from build123d import *

# Parameters (mm, degrees)
SKETCH_1_W               = 64
SKETCH_1_H               = 34
SKETCH_1_W_2             = 60
SKETCH_1_H_2             = 30
EXTRUDE_1_DEPTH          = 28
SKETCH_1_2_W             = 60
SKETCH_1_2_H             = 30
EXTRUDE_1_2_DEPTH        = 2
FILLET_3_R               = 2.5
CUT_EXTRUDE_6_DEPTH      = 55.442630355
CUT_EXTRUDE_6_DEPTH_BACK = 55.442630355
FILLET_4_R               = 10
SKETCH_8_W               = 30
SKETCH_8_H               = 4.631369762
CUT_EXTRUDE_7_DEPTH      = 71.121323433
CUT_EXTRUDE_9_DEPTH      = 45.598206242
CUT_EXTRUDE_9_DEPTH_BACK = 45.598206242
SKETCH_9_R               = 2


with BuildPart() as part:
    # Эскиз1 → Extrude 1 (new body)
    with BuildSketch(Plane(origin=(0, 0, 0), x_dir=(1, 0, 0), z_dir=(0, 1, 0))):
        Rectangle(SKETCH_1_W, SKETCH_1_H)
        Rectangle(SKETCH_1_W_2, SKETCH_1_H_2, mode=Mode.SUBTRACT)
    extrude(amount=EXTRUDE_1_DEPTH)

    # Эскиз1<2> → Extrude 1 2 (add)
    with BuildSketch(Plane(origin=(0, 0, 0), x_dir=(1, 0, 0), z_dir=(0, 1, 0))):
        Rectangle(SKETCH_1_2_W, SKETCH_1_2_H)
    extrude(amount=EXTRUDE_1_2_DEPTH)

    # Скругление3
    fillet_3_edges = [part.edges().sort_by_distance(p)[0] for p in [
        (-30, 15, -15),
        (-30, 15, 15),
        (-32, 14, -17),
        (-32, 14, 17),
    ]]
    fillet(fillet_3_edges, radius=FILLET_3_R)

    # Эскиз3 → Вырез-Вытянуть6 (cut, two sides: drawn at the far end of the back side and taken through both)
    with BuildSketch(Plane.XY.offset(17).offset(-CUT_EXTRUDE_6_DEPTH_BACK)):
        Polygon((-13, 28), (32, 7), (32, 28), align=None)
    extrude(amount=CUT_EXTRUDE_6_DEPTH + CUT_EXTRUDE_6_DEPTH_BACK, mode=Mode.SUBTRACT)

    # Скругление4
    # the kernel refuses this fillet: 10 mm, written as the material it takes off along each edge
    with BuildSketch(Plane(origin=(32, 7, -32.921575595), x_dir=(0, -1, 0), z_dir=(0, 0, 1))) as fillet_4_piece_1:
        with BuildLine():
            CenterArc((FILLET_4_R * 0.636863023816, -FILLET_4_R), FILLET_4_R, 90, 64.983106522)
            Line((-FILLET_4_R * 0.269320116179, -FILLET_4_R * 0.577114534669), (0, 0))
            Line((0, 0), (FILLET_4_R * 0.636863023816, 0))
        make_face()
    extrude(amount=65.843151191, mode=Mode.SUBTRACT)
    with BuildSketch(Plane(origin=(-13, 28, 22.546233419), x_dir=(0.9061831399952657, -0.4228854653311234, 0), z_dir=(0, 0, -1)), Plane(origin=(-13, 28, -9.453766581), x_dir=(0.9061831399952657, -0.4228854653311234, 0), z_dir=(0, 0, -1))) as fillet_4_piece_2:
        with BuildLine():
            CenterArc((FILLET_4_R * 0.22184933675, FILLET_4_R), FILLET_4_R, 244.983106522, 25.016893478)
            Line((-FILLET_4_R * 0.201036128582, FILLET_4_R * 0.0938168600047), (0, 0))
            Line((0, 0), (FILLET_4_R * 0.22184933675, 0))
        make_face()
    extrude(amount=13.092466837, mode=Mode.SUBTRACT)

    # Эскиз8 → Вырез-Вытянуть7 (cut, through all)
    with BuildSketch(Plane.ZY.offset(-30)):
        with Locations((0, 4.315684881)):
            Rectangle(SKETCH_8_W, SKETCH_8_H)
    extrude(amount=-CUT_EXTRUDE_7_DEPTH, mode=Mode.SUBTRACT)

    # Эскиз9 → Вырез-Вытянуть9 (cut, two sides: drawn at the far end of the back side and taken through both)
    with BuildSketch(Plane(origin=(0, 2, 0), x_dir=(1, 0, 0), z_dir=(0, 1, 0)).offset(-CUT_EXTRUDE_9_DEPTH_BACK)):
        with Locations(Location((-22.5, -10, 0), (0, 0, 270))):
            Circle(SKETCH_9_R)
        with Locations(Location((-22.5, 10, 0), (0, 0, 270))):
            Circle(SKETCH_9_R)
        with Locations(Location((22.5, 10, 0), (0, 0, 270))):
            Circle(SKETCH_9_R)
        with Locations(Location((22.5, -10, 0), (0, 0, 270))):
            Circle(SKETCH_9_R)
    extrude(amount=CUT_EXTRUDE_9_DEPTH + CUT_EXTRUDE_9_DEPTH_BACK, mode=Mode.SUBTRACT)


solid = part.part
Part model, mm, in its own coordinate system. A direction names the side the tool comes from. Round coordinates to 2 decimals unless told otherwise and drop trailing zeros. Write each loop counter-clockwise with the first axis right and the second up, starting at its lowest first coordinate (ties: lowest second). Pieces come first, ordered by that corner, then holes. Notation, with made-up numbers: M 41,61.5 L 96,61.5 A15 cw 96,70.5 Z; hole C 40,66 d10. An arc over 180 degrees is marked long. Return JSON: item names as keys, results as strings. Group by question number.
(1) Saw through at B-B on x = -22.5. Write the cut outline in (y, z), then the cut area to 3 significant figures.
(2) Saw through at D-D on y = 15.75. Write the cut outline in (x, z).
(3) Pin check, flat tip, straight feed: pin 1 Ø15 at (x, z) = (2.5, -4) entering from +Y. Stop position of the tip, or through.
(4) Saw through at C-C on z = -5.5. Write the cut outline in (x, y), then the cut area to 3 significant figures.
(5) Which spindle directions (+Z, -Z, +X, -X, +Y, -Y) get a long thin tool onto all of the face, cutting with end or side? Do faces 1 (the face through (-30.5, 28, -0.1)), 2 (the face through (-29.248, 15.182, -14.287)). Say none if no direction does.
(6) Drill centre lines: probe 1 along X at (y, z) = (0.4, 10); probe 2 along Z at (x, y) = (-22.5, 1.05); probe 3 along Z at (x, y) = (3, 19.5). Where is each one in solid material? Low to high.
(7) Saw through at A-A on z = -10. Write the cut outline in (x, y), then the cut area to 3 significant figures.
(8) Two-plate mould, pull along Z, no slides. Class faces 3 (the face through (-13.08, 27.77, -15.99)), 4 (the face through (-31.287, 14.196, 16.248)), 5 (the face through (-20.517, 0.986, 9.74)): +Z half, -Z half, draft (parallel to the pull), parting line (faces both ways), or undercut.
Returned:
{
 "1": {"outline": "M 0,-17 L 28,-17 L 28,-15 L 2,-15 L 2,-12 L 0,-12 Z; M 0,-8 L 2,-8 L 2,8 L 0,8 Z; M 0,12 L 2,12 L 2,15 L 28,15 L 28,17 L 0,17 Z", "area": "156 mm²"},
 "2": {"outline": "M -32,-14.5 A2.5 ccw -29.5,-17 L 13.25,-17 L 13.25,-15 L -27.5,-15 A2.5 cw -30,-12.5 L -30,12.5 A2.5 cw -27.5,15 L 13.25,15 L 13.25,17 L -29.5,17 A2.5 ccw -32,14.5 Z"},
 "3": {"pin 1": "y = 2"},
 "4": {"outline": "M -32,0 L 32,0 L 32,0.63 A10 ccw 31.91,2 L -30,2 L -30,28 L -32,28 Z", "area": "180 mm²"},
 "5": {"face 1": "+Z, -Z, +X, -X, +Y", "face 2": "+X, +Y"},
 "6": {"probe 1": "-32 to -24.5, -20.5 to 20.5, 24.5 to 32", "probe 2": "-17 to -12, -8 to 8, 12 to 17", "probe 3": "-17 to -15, 15 to 17"},
 "7": {"outline": "M -32,0 L -24.5,0 L -24.5,2 L -30,2 L -30,28 L -32,28 Z; M -20.5,0 L 20.5,0 L 20.5,2 L -20.5,2 Z; M 24.5,0 L 32,0 L 32,0.63 A10 ccw 31.91,2 L 24.5,2 Z", "area": "164 mm²"},
 "8": {"face 3": "draft", "face 4": "+Z half", "face 5": "undercut"}
}
